The figure shows three views and two pictorial views of one solid part (mm, origin at its lowest corner). Answer the questions. Give positions to 0.01 mm unless a question says otherwise; leave off trailing zeros. Order: outer loops, then holes, each group sorted by start corner. A loop starts at its lowest first (then second) coordinate and runs counter-clockwise, first axis right, second up. Notation, with made-up numbers: (10, 72) -> (55, 72) arc R27 ccw to (55, 103) -> close; hole circle Ø3 at (-36, 20). An arc over 180 degrees is marked (long way). Use one line per item in the form item = value.
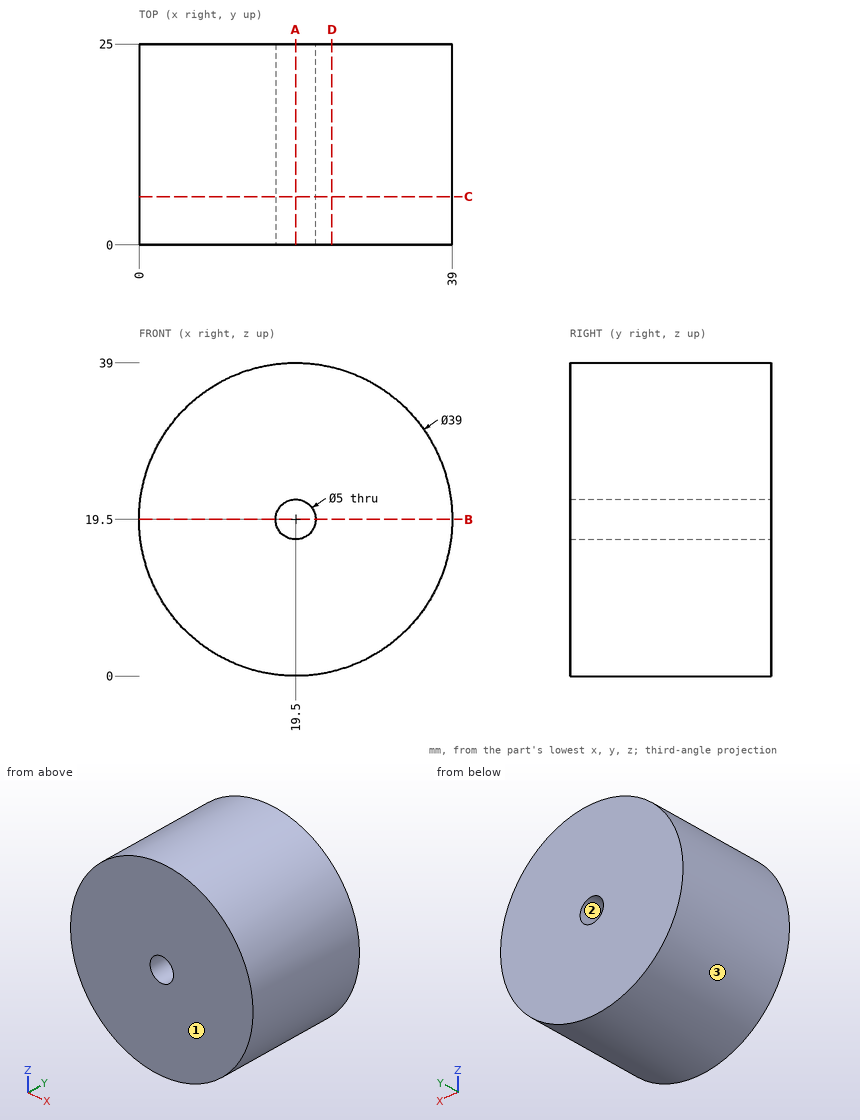
Item 1: The part is cut by section C-C on y = 6. Give the vertices of the cut face in (x, z), and give its area (3 significant figures).
Checks:
outline = circle Ø39 at (19.5, 19.5); hole circle Ø5 at (19.5, 19.5)
area = 1,170 mm²
Item 2: Straight lines are drawn through the part: L1, parallel to Z at x = 30.5, y = 11; L2, parallel to Z at x = 34, y = 4.75; L3, parallel to X at y = 23.75, z = 37. For each, find the intervals that lie inside material, in ascending order. Write a range as from..to.
Checks:
L1 = 3.4..35.6
L2 = 6.46..32.54
L3 = 10.9..28.1
Item 3: The part is cut by section B-B on z = 19.5. Give the vertices of the cut face in (x, y), and give its area (3 significant figures).
Checks:
outline = (0, 0) -> (17, 0) -> (17, 25) -> (0, 25) -> close; (22, 0) -> (39, 0) -> (39, 25) -> (22, 25) -> close
area = 850 mm²
Item 4: The part is cut by section A-A on x = 19.5. Give the vertices of the cut face in (y, z), and give its area (3 significant figures).
Checks:
outline = (0, 0) -> (25, 0) -> (25, 17) -> (0, 17) -> close; (0, 22) -> (25, 22) -> (25, 39) -> (0, 39) -> close
area = 850 mm²
Item 5: Determine the mould class of the marked faces 1, 2 and 3 for opening direction Z: +Z half, -Z half, draft (parallel to the pull), parting line (faces both ways), or undercut.
Checks:
face_1 = draft
face_2 = undercut
face_3 = parting line
Item 6: Given pin 1 Ø1 at (x, z) = (30.5, 22) entering from -Y; pin 2 Ø6 at (x, y) = (28.5, 7) entering from +Z; pin 3 Ø3 at (x, y) = (7.5, 12.5) entering from -Z; pin 4 Ø2 at (x, y) = (9.5, 12) entering from -Z, each flat-ended and moving along its own axis, determine where each tip first touches the part or whether it passes through.
Checks:
pin_1 = 0
pin_2 = 38.05
pin_3 = 3.07
pin_4 = 2.2
Item 7: The part is cut by section D-D on x = 24. Give the vertices of the cut face in (y, z), and give its area (3 significant figures).
Checks:
outline = (0, 0.53) -> (25, 0.53) -> (25, 38.47) -> (0, 38.47) -> close
area = 949 mm²
